Geometry: see drawing. Coordinates: mm, zero at the bounding-box minimum. Round coordinates to 2 decimals unless told otherwise and drop trailing zeros. Loops run counter-clockwise (first coordinate to the right, second up) from the corner with the lowest first, then second, coordinate; pieces in that order, holes last. Notation, with made-up numbers: M -25.5,-32.5 L 21.5,-32.5 A15 cw 21.5,-27.5 Z; hole C 30,89.5 d2. An arc over 180 degrees is marked long. Answer as a JSON object with one key per item and string values.
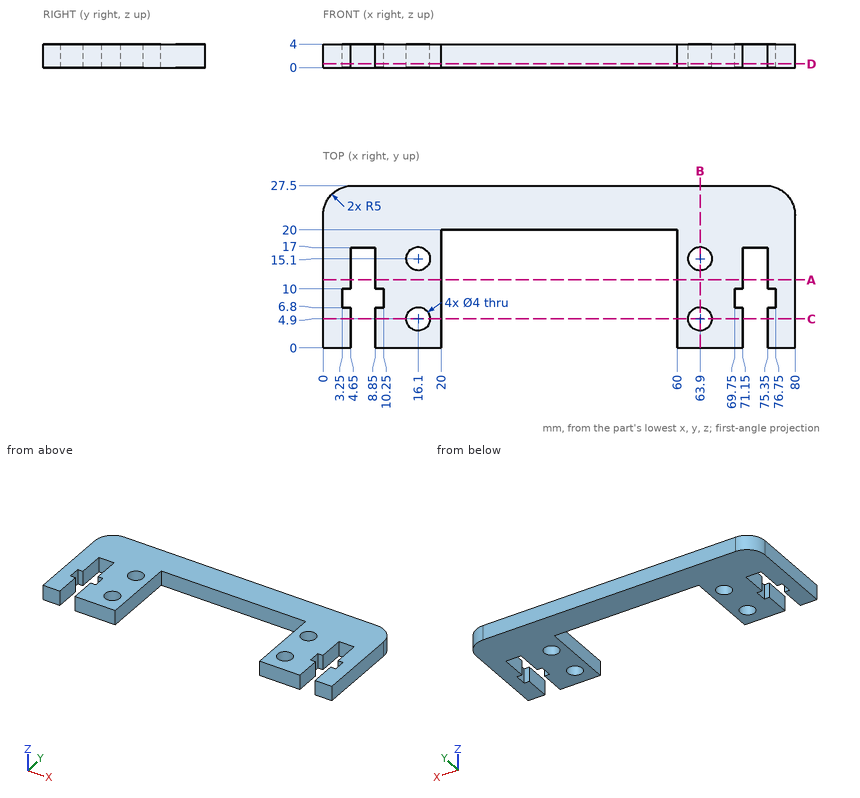
1) Ray query, line 1 (Y direction, x = 63.9, z = 1.45); line 2 (X direction, y = 19.25, z = 1); line 3 (X direction, y = 5.5, z = 0.55). Return the intervals inside material, ascending.
Results:
{"line 1": "0 to 2.9, 6.9 to 13.1, 17.1 to 27.5", "line 2": "0 to 20, 60 to 80", "line 3": "0 to 4.65, 8.85 to 14.19, 18.01 to 20, 60 to 61.99, 65.81 to 71.15, 75.35 to 80"}
2) Section query C-C (y = 4.9). Return the cut outline in (x, z), and give its area (3 significant figures).
Results:
{"outline": "M 0,0 L 4.65,0 L 4.65,4 L 0,4 Z; M 8.85,0 L 14.1,0 L 14.1,4 L 8.85,4 Z; M 18.1,0 L 20,0 L 20,4 L 18.1,4 Z; M 60,0 L 61.9,0 L 61.9,4 L 60,4 Z; M 65.9,0 L 71.15,0 L 71.15,4 L 65.9,4 Z; M 75.35,0 L 80,0 L 80,4 L 75.35,4 Z", "area": "94.4 mm2"}
3) Section query D-D (z = 0.65). Count the separate pieces of the cut face and the enclosed holes in it, and give its area (3 significant figures).
Results:
{"separate pieces": "1", "enclosed holes": "4", "area": "1,180 mm2"}
4) Pin query (flat end, axial travel): P1, Ø5, axis at x = 63.9, y = 4.9, coming from the +Z side; P2, Ø2, axis at x = 51.5, z = 0.5, coming from the -Y side; P3, Ø1.1, axis at x = 3.5, z = 3, coming from the +Y side; P4, Ø1.2, axis at x = 6.5, z = 2.5, coming from the -Y side. Return the tip coordinate at first contact, or that it passes through.
Results:
{"P1": "z = 4", "P2": "y = 20", "P3": "y = 27.41", "P4": "y = 17"}
5) Section query B-B (x = 63.9). Return the cut outline in (y, z), and give its area (3 significant figures).
Results:
{"outline": "M 0,0 L 2.9,0 L 2.9,4 L 0,4 Z; M 6.9,0 L 13.1,0 L 13.1,4 L 6.9,4 Z; M 17.1,0 L 27.5,0 L 27.5,4 L 17.1,4 Z", "area": "78.0 mm2"}
6) Section query A-A (y = 11.5). Return the cut outline in (x, z), and give its area (3 significant figures).
Results:
{"outline": "M 0,0 L 4.65,0 L 4.65,4 L 0,4 Z; M 8.85,0 L 20,0 L 20,4 L 8.85,4 Z; M 60,0 L 71.15,0 L 71.15,4 L 60,4 Z; M 75.35,0 L 80,0 L 80,4 L 75.35,4 Z", "area": "126 mm2"}
